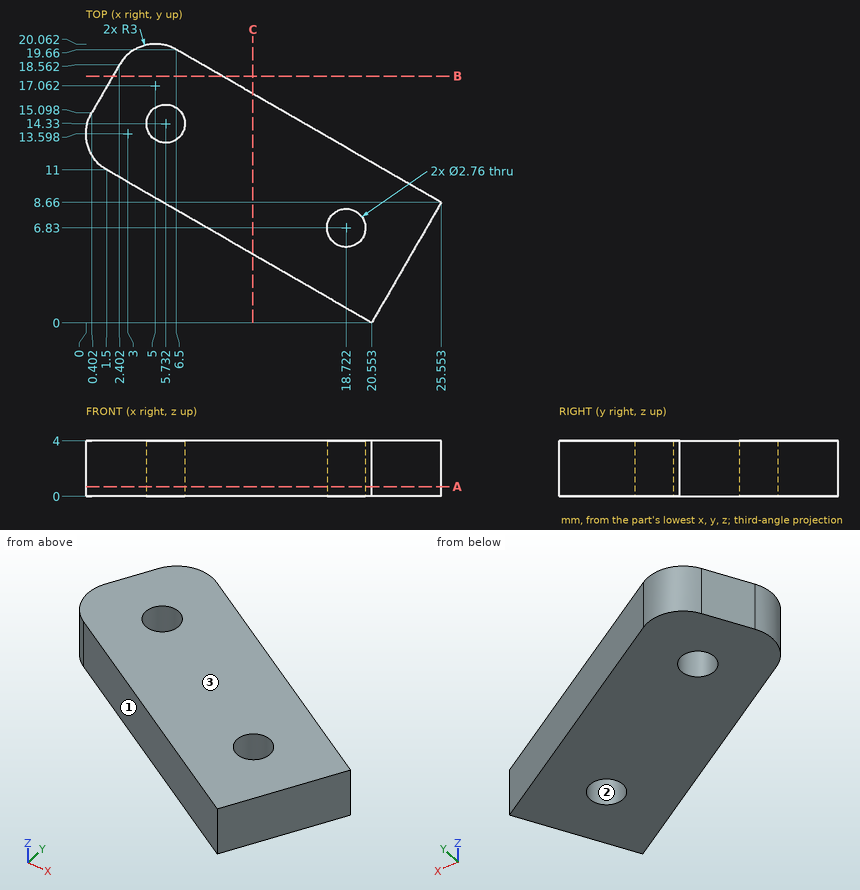
Input: dimensioned drawing with shaded views. Units: mm. Origin: part minimum x, y, z. Coordinates: 2 decimals unless noted, no trailing zeros. Order: outer loops, then holes, each group sorted by start corner. A loop starts at its lowest first (then second) coordinate and runs counter-clockwise, first axis right, second up. Notation, with made-up numbers: (-31, 17.25) -> (-15, 17.25) arc R26 cw to (-15, 40.25) -> close; hole circle Ø10 at (-26.5, 82). An arc over 180 degrees is marked (long way). Answer in a Markdown table with one row per item.
Item 1: Contact query for flat-ended pins moving along their axis: P1, Ø3, axis at x = 18.72, y = 6.83, coming from the +Z side; P2, Ø1.5, axis at x = 4.5, z = 2.5, coming from the -Y side (1 decimal); P3, Ø1, axis at x = 3.5, y = 8.5, coming from the -Z side. Output: stop coordinate, or through.
Return value:
| item | result |
|---|---|
| P1 | stops at z = 4 |
| P2 | stops at y = 8.8 |
| P3 | passes through |
Item 2: Section A-A on z = 0.7. Output: boundary loops of the cut face in (x, y).
Return value:
| item | result |
|---|---|
| outline | (0.4, 15.1) arc R3 ccw to (1.5, 11) -> (20.55, 0) -> (25.55, 8.66) -> (6.5, 19.66) arc R3 ccw to (2.4, 18.56) -> close; hole circle Ø2.76 at (5.73, 14.33); hole circle Ø2.76 at (18.72, 6.83) |
Item 3: Section B-B on y = 17.75. Output: boundary loops of the cut face in (x, z).
Return value:
| item | result |
|---|---|
| outline | (1.93, 0) -> (9.81, 0) -> (9.81, 4) -> (1.93, 4) -> close |
Item 4: Draft query along X for the marked faces 1, 2 and 3. Return one class per face: released by +X, released by -X, zero draft, split by the parting line, or undercut.
Return value:
| item | result |
|---|---|
| face 1 | released by -X |
| face 2 | undercut |
| face 3 | zero draft |
Item 5: Section C-C on x = 12. Output: boundary loops of the cut face in (y, z) (1 decimal), plus the area to 3 significant figures.
Return value:
| item | result |
|---|---|
| outline | (4.9, 0) -> (16.5, 0) -> (16.5, 4) -> (4.9, 4) -> close |
| area | 46.2 mm² |
Item 6: Ray query, L1, parallel to Y at x = 18, z = 0.7 (1 decimal); L2, parallel to X at y = 6.5, z = 0.95 (1 decimal); L3, parallel to Y at x = 17.5, z = 2.9 (1 decimal). Return the intervals inside material, ascending.
Return value:
| item | result |
|---|---|
| L1 | y = 1.5 to 5.7, 8 to 13 |
| L2 | x = 9.3 to 17.4, 20.1 to 24.3 |
| L3 | y = 1.8 to 6.2, 7.5 to 13.3 |
